from build123d import *

# Parameters (mm, degrees)
F1_DEPTH  = 8
F3_DEPTH  = 3
F7_DEPTH  = 3
F8_R      = 2.1
F9_DEPTH  = 5
F13_DEPTH = 25


with BuildPart() as f1:
    # F0 (on Front) → F1 (new body)
    with BuildSketch(Plane.XZ):
        with BuildLine():
            Line((-87, -32), (87, -32))
            ThreePointArc((87, -32), (91.949747, -29.949747), (94, -25))
            Line((94, -25), (94, 25))
            ThreePointArc((94, 25), (91.949747, 29.949747), (87, 32))
            Line((87, 32), (-87, 32))
            ThreePointArc((-87, 32), (-91.949747, 29.949747), (-94, 25))
            Line((-94, 25), (-94, -25))
            ThreePointArc((-94, -25), (-91.949747, -29.949747), (-87, -32))
        make_face()
    extrude(amount=F1_DEPTH)

    # F2 (on face) → F3 (cut)
    with BuildSketch(Plane.XZ.offset(8)):
        with BuildLine():
            Line((87, 30), (-87, 30))
            ThreePointArc((-87, 30), (-90.535534, 28.535534), (-92, 25))
            Line((-92, 25), (-92, -25))
            ThreePointArc((-92, -25), (-90.535534, -28.535534), (-87, -30))
            Line((-87, -30), (87, -30))
            ThreePointArc((87, -30), (90.535534, -28.535534), (92, -25))
            Line((92, -25), (92, 25))
            ThreePointArc((92, 25), (90.535534, 28.535534), (87, 30))
        make_face()
    extrude(amount=-F3_DEPTH, mode=Mode.SUBTRACT)

    # F6 (on face) → F7 (cut)
    with BuildSketch(Plane.XZ.offset(5)):
        Polygon((55.669873, -20), (57.834936, -23.75), (62.165064, -23.75), (64.330127, -20), (62.165064, -16.25), (57.834936, -16.25), align=None)
        Polygon((78.669873, 20), (80.834936, 16.25), (85.165064, 16.25), (87.330127, 20), (85.165064, 23.75), (80.834936, 23.75), align=None)
        Polygon((-64.330127, -20), (-62.165064, -23.75), (-57.834936, -23.75), (-55.669873, -20), (-57.834936, -16.25), (-62.165064, -16.25), align=None)
        Polygon((-87.330127, 20), (-85.165064, 16.25), (-80.834936, 16.25), (-78.669873, 20), (-80.834936, 23.75), (-85.165064, 23.75), align=None)
    extrude(amount=-F7_DEPTH, mode=Mode.SUBTRACT)

    # F8 (on face) → F9 (cut, through all)
    with BuildSketch(Plane.XZ.offset(5)):
        with Locations((-83, 20)):
            Circle(F8_R)
        with Locations((-60, -20)):
            Circle(F8_R)
        with Locations((83, 20)):
            Circle(F8_R)
        with Locations((60, -20)):
            Circle(F8_R)
    extrude(amount=-F9_DEPTH, mode=Mode.SUBTRACT)

    # F12 (on face) → F13 (cut)
    with BuildSketch(Plane.XZ.offset(5)):
        with BuildLine():
            ThreePointArc((79, -13), (79.292893, -13.707107), (80, -14))
            Line((80, -14), (83, -14))
            ThreePointArc((83, -14), (83.707107, -13.707107), (84, -13))
            Line((84, -13), (84, 10))
            ThreePointArc((84, 10), (83.707107, 10.707107), (83, 11))
            Line((83, 11), (80, 11))
            ThreePointArc((80, 11), (79.292893, 10.707107), (79, 10))
            Line((79, 10), (79, -13))
        make_face()
    extrude(amount=-F13_DEPTH, mode=Mode.SUBTRACT)


solid = f1.part
Verification items for the finished model (mm, model axes). A direction names the side the tool comes from. Round coordinates to 2 decimals unless told otherwise and drop trailing zeros. Write each loop counter-clockwise with the first axis right and the second up, starting at its lowest first coordinate (ties: lowest second). Pieces come first, ordered by that corner, then holes.
(1) Mould release check, pull along X, two halves, no side actions. Record for faces 4 (the flat face through (1, -4, 32)), 5 (the flat face through (56.768, -3.521, -18.099)), 6 (the flat face through (60, -4, -16.25)), 7 (the cylindrical face through (91.9, -3.9, -30)): pulls with the +X half, pulls with the -X half, needs draft (parallel to the pull), parting line crosses it, or undercut.
Returned:
face 4: needs draft
face 5: undercut
face 6: undercut
face 7: pulls with the +X half
(2) Section check A-A (x = -60). Enter the section's corners in (y, z).
Returned:
outline: (-8, -32) - (0, -32) - (0, -22.1) - (-2, -22.1) - (-2, -23.75) - (-5, -23.75) - (-5, -30) - (-8, -30) - close; (-8, 30) - (-5, 30) - (-5, -16.25) - (-2, -16.25) - (-2, -17.9) - (0, -17.9) - (0, 32) - (-8, 32) - close
(3) Access from +Z, -Z, +X, -X, +Y, -Y to the whole of each face (thin tool, end or side, straight path). Record for faces 1 (the flat face through (56.74, -3.52, -21.85)), 2 (the flat face through (81, -3, -14)), 3 (the cylindrical face through (92, -3.9, 29.9)).
Returned:
face 1: -Y
face 2: +Y, -Y
face 3: +Z, +X, +Y, -Y
(4) Depth check by flat-ended pin: pin 1 Ø6 at (x, z) = (6.5, 10.5) entering from +Y; pin 2 Ø4 at (x, z) = (-43.5, -4) entering from -Y; pin 3 Ø4 at (x, z) = (-83, 20) entering from -Y; pin 4 Ø5.5 at (x, z) = (60, -20) entering from -Y. Enter the tip coordinate at first touch or a pass-through.
Returned:
pin 1: stops at y = 0
pin 2: stops at y = -5
pin 3: passes through
pin 4: stops at y = -2
(5) Section check C-C (y = -3.5). Give the number of separate pieces and of enclosed holes in the cut face, plus the area to 3 significant figures.
Returned:
separate pieces: 1
enclosed holes: 5
area: 11,700 mm2
(6) Material ranges on line 1 (X direction, y = -6.5, z = 14); line 2 (Z direction, x = -60, y = -1.6); line 3 (Z direction, x = 83, y = -1), recorded low to high.
Returned:
line 1: x = -94 to -92, 92 to 94
line 2: z = -32 to -22.1, -17.9 to 32
line 3: z = -32 to -14, 11 to 17.9, 22.1 to 32
(7) Section check B-B (z = 14.5). Enter the section's corners in (x, y).
Returned:
outline: (-94, -8) - (-92, -8) - (-92, -5) - (92, -5) - (92, -8) - (94, -8) - (94, 0) - (-94, 0) - close
